from build123d import *

# Parameters (mm, degrees)
BOSS_EXTRU_1_DEPTH      = 60
ESQUISSE2_W             = 12
ESQUISSE2_H             = 30
ENL_V_MAT_EXTRU_1_DEPTH = 72.119617547


with BuildPart() as part:
    # Esquisse1 → Boss.-Extru.1 (new body)
    with BuildSketch(Plane.XY):
        with BuildLine():
            Line((-27, 0), (-25, 0))
            ThreePointArc((-25, 0), (0, -25), (25, 0))
            Line((25, 0), (27, 0))
            ThreePointArc((27, 0), (0, -27), (-27, 0))
        make_face()
    extrude(amount=BOSS_EXTRU_1_DEPTH)

    # Esquisse2 → Enlèv. mat.-Extru.1 (cut, through all)
    with BuildSketch(Plane(origin=(0, 0, 0), x_dir=(1, 0, 0), z_dir=(0, 1, 0))):
        with Locations((0, -36.544954045)):
            Rectangle(ESQUISSE2_W, ESQUISSE2_H)
    extrude(amount=-ENL_V_MAT_EXTRU_1_DEPTH, mode=Mode.SUBTRACT)


solid = part.part
Geometry check sheet. Reference: the model listing, model coordinates, mm. A direction names the side the tool comes from. Give positions to 0.01 mm unless a question says otherwise; leave off trailing zeros. Order: outer loops, then holes, each group sorted by start corner. A loop starts at its lowest first (then second) coordinate and runs counter-clockwise, first axis right, second up.
1) Tool access check on faces 1 (the flat face through (-26, 0, 30)), 2 (the flat face through (6, -25, 37)). Record the directions out of +Z, -Z, +X, -X, +Y, -Y that give a thin tool (end or side, any length) a straight path to the whole face; none if there is none.
Results are:
face 1: +Z, -Z, +X, -X, +Y
face 2: +Y, -Y
2) Material ranges on probe 1 along X at (y, z) = (-18.5, 18); probe 2 along X at (y, z) = (-22.25, 49); probe 3 along Y at (x, z) = (-15.5, 42), recorded low to high.
Results are:
probe 1: x = -19.67 to -16.82, 16.82 to 19.67
probe 2: x = -15.3 to -11.4, 11.4 to 15.3
probe 3: y = -22.11 to -19.62
3) Cross-section at A-A (z = 30). Record the boundary of the cut face in (x, y).
Results are:
outline: (-27, 0) arc R27 ccw to (-6, -26.32) - (-6, -24.27) arc R25 cw to (-25, 0) - close; (6, -26.32) arc R27 ccw to (27, 0) - (25, 0) arc R25 cw to (6, -24.27) - close
4) Draft check along X on faces 3 (the cylindrical face through (8.032, -23.675, 29.58)), 4 (the flat face through (0, -26, 51.545)), 5 (the cylindrical face through (9.79, -25.163, 29.58)), 6 (the flat face through (0.1, -25.4, 0)). Enter one of: released by +X, released by -X, zero draft, split by the parting line, or undercut.
Results are:
face 3: undercut
face 4: undercut
face 5: split by the parting line
face 6: zero draft
5) Gauge pin test, flat ends, axial feed: pin 1 (1 mm diameter, centred on y = -25, z = 35.5, fed in from -X); pin 2 (6 mm diameter, centred on y = -11.5, z = 22.5, fed in from -X); pin 3 (1.5 mm diameter, centred on y = -13, z = 40.5, fed in from +X). Record the tip position at first contact, or that the pin passes through.
Results are:
pin 1: stops at x = -11.35
pin 2: stops at x = -25.63
pin 3: stops at x = 24.06
6) Cross-section at D-D (x = 7). Record the boundary of the cut face in (y, z).
Results are:
outline: (-26.08, 0) - (-24, 0) - (-24, 60) - (-26.08, 60) - close
7) Cross-section at B-B (x = 0). Record the boundary of the cut face in (y, z).
Results are:
outline: (-27, 0) - (-25, 0) - (-25, 21.54) - (-27, 21.54) - close; (-27, 51.54) - (-25, 51.54) - (-25, 60) - (-27, 60) - close
8) Cross-section at C-C (z = 13). Record the boundary of the cut face in (x, y), then the cut area to 3 significant figures.
Results are:
outline: (-27, 0) arc R27 ccw to (27, 0) - (25, 0) arc R25 cw to (-25, 0) - close
area: 163 mm2
